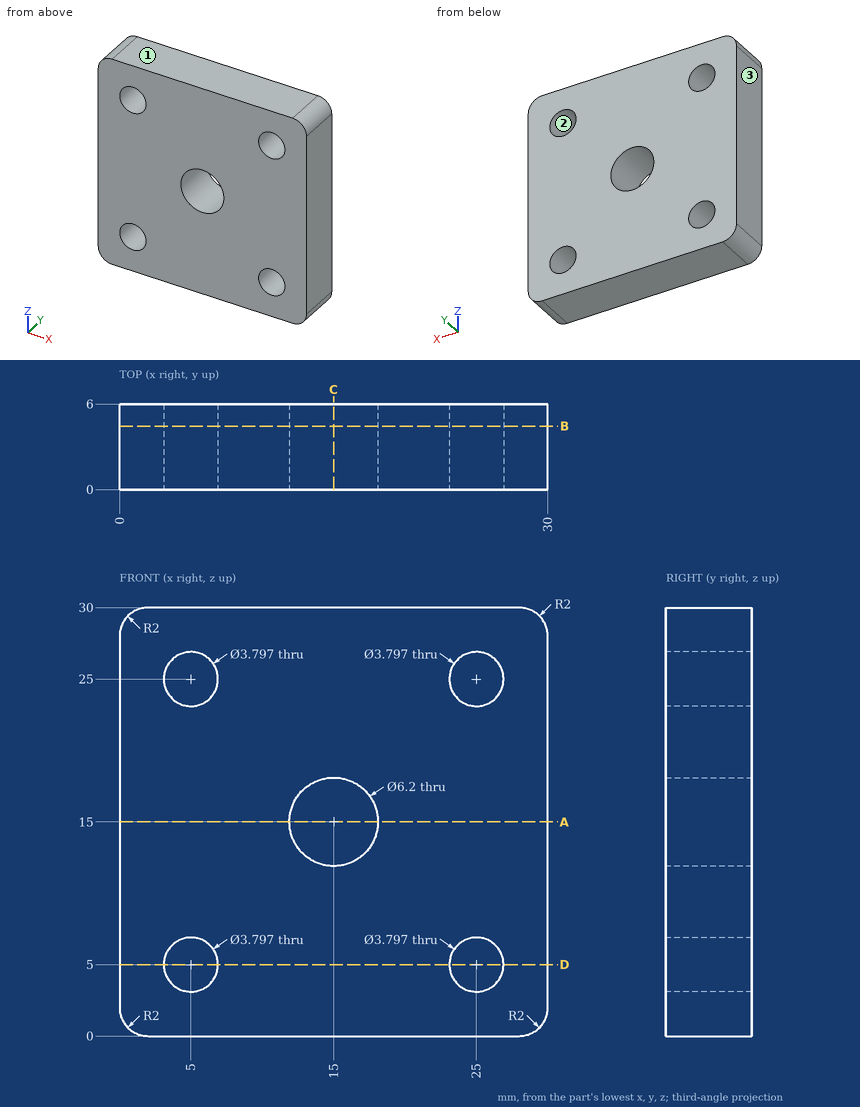
Verification items for this drawing (mm, ordinates from the low corner). Round coordinates to 2 decimals unless told otherwise and drop trailing zeros. Write each loop counter-clockwise with the first axis right and the second up, starting at its lowest first coordinate (ties: lowest second). Pieces come first, ordered by that corner, then holes. Notation, with made-up numbers: (10.5, -5) - (28.5, -5) arc R28 ccw to (28.5, 28) - close; hole circle Ø3 at (17, -26.5). An arc over 180 degrees is marked (long way). Answer as a JSON object with one key per item and string values. Group by question number.
Q1. Thickness scan on line 1 (X direction, y = 2.15, z = 25); line 2 (X direction, y = 1.8, z = 25.75) (1 decimal). Record the ranges inside material, lowest first.
Q2. Section check D-D, the plane z = 5. Enter the section's corners in (x, y).
Q3. Mould release check, pull along X, two halves, no side actions. Record for the marked faces 1, 2 and 3: released by +X, released by -X, zero draft, split by the parting line, or undercut.
Q4. Section check B-B, the plane y = 4.45. Enter the section's corners in (x, z).
Q5. Section check C-C, the plane x = 15. Enter the section's corners in (y, z), plus the area to 3 significant figures.
Q6. Section check A-A, the plane z = 15. Enter the section's corners in (x, y).
Found:
{
 "1": {"line 1": "x = 0 to 3.1, 6.9 to 23.1, 26.9 to 30", "line 2": "x = 0 to 3.3, 6.7 to 23.3, 26.7 to 30"},
 "2": {"outline": "(0, 0) - (3.1, 0) - (3.1, 6) - (0, 6) - close; (6.9, 0) - (23.1, 0) - (23.1, 6) - (6.9, 6) - close; (26.9, 0) - (30, 0) - (30, 6) - (26.9, 6) - close"},
 "3": {"face 1": "zero draft", "face 2": "undercut", "face 3": "released by -X"},
 "4": {"outline": "(0, 2) arc R2 ccw to (2, 0) - (28, 0) arc R2 ccw to (30, 2) - (30, 28) arc R2 ccw to (28, 30) - (2, 30) arc R2 ccw to (0, 28) - close; hole circle Ø3.8 at (5, 5); hole circle Ø3.8 at (5, 25); hole circle Ø6.2 at (15, 15); hole circle Ø3.8 at (25, 5); hole circle Ø3.8 at (25, 25)"},
 "5": {"outline": "(0, 0) - (6, 0) - (6, 11.9) - (0, 11.9) - close; (0, 18.1) - (6, 18.1) - (6, 30) - (0, 30) - close", "area": "143 mm^2"},
 "6": {"outline": "(0, 0) - (11.9, 0) - (11.9, 6) - (0, 6) - close; (18.1, 0) - (30, 0) - (30, 6) - (18.1, 6) - close"}
}
